The listing builds one solid part. Answer for the finished solid, in the listing's coordinates (mm). Face numbers are marked on the shaded views. A direction names the side the tool comes from. Give positions to 0.01 mm unless a question says otherwise; leave off trailing zeros. Order: outer loops, then holes, each group sorted by start corner. A loop starts at its lowest first (then second) coordinate and runs counter-clockwise, first axis right, second up. Notation, with made-up numbers: (66, 75.5) - (116, 75.5) arc R19 cw to (116, 83.5) - close; hole circle Ø5 at (42, 29). An arc over 180 degrees is marked (long way). Answer as CSV lines item,"result". Start each with the question number.
1. Section D-D on y = 21.75 is taken. Give the vertices of the cut face in (x, z).
2. Section A-A on z = -1 is taken. Give the vertices of the cut face in (x, y).
3. Section B-B on x = 15 is taken. Give the vertices of the cut face in (y, z), and give its area (3 significant figures).
4. Section C-C on z = -10 is taken. Give the vertices of the cut face in (x, y), and give its area (3 significant figures).
5. Flat-ended cylindrical pins translate along their axes: pin 1 (2 mm diameter, centred on x = 15, z = -10, fed in from -Y); pin 2 (1 mm diameter, centred on x = 12, y = 7, fed in from +Z); pin 3 (6 mm diameter, centred on x = 15.5, y = 12.5, fed in from -Z). Find the tip coordinate at first contact, or state that the pin passes through.
6. Consider line 1 along X through (y, z) = (7.35, -10); line 2 along Y through (x, z) = (10.75, -4); line 3 along Z through (x, y) = (15, 23.05). Determine where each line is inside the solid, lowest interval first. Write a range as [from, to].
7. Which of the six approach directions +Z, -Z, +X, -X, +Y, -Y give full straight-line access (tool end or side, diameter ignored) to the marked faces 5 and 6?
8. Determine the mould class of the marked faces 1, 2, 3 and 4 for opening direction Y: +Y half, -Y half, draft (parallel to the pull), parting line (faces both ways), or undercut.
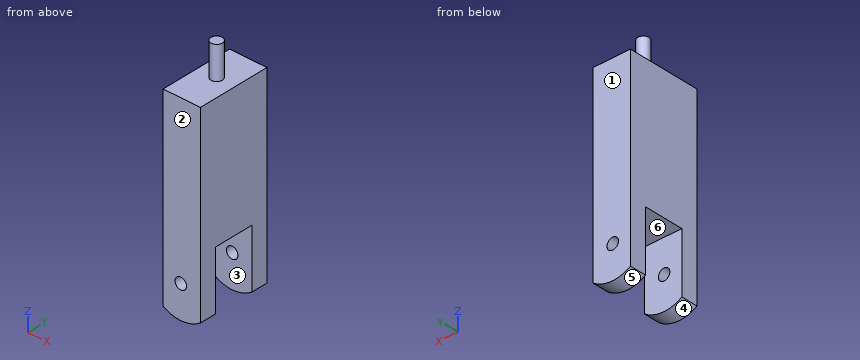
from build123d import *

# Parameters (mm, degrees)
SKETCH3_W            = 30
SKETCH3_H            = 30
BOSS_EXTRUDE1_DEPTH  = 40
CUT_EXTRUDE4_START   = -40
CUT_EXTRUDE4_DEPTH   = 99.309518948
MIRROR5_START        = -40
MIRROR5_COPY_1_DEPTH = 99.309518948
SKETCH9_R            = 1.75
BOSS_EXTRUDE2_DEPTH  = 30
CUT_EXTRUDE5_DEPTH   = 30
SKETCH11_W           = 20
SKETCH11_H           = 12.2
CUT_EXTRUDE6_DEPTH   = 44.5
SKETCH12_R           = 1.75
BOSS_EXTRUDE3_DEPTH  = 10
CUT_EXTRUDE13_DEPTH  = 67
SKETCH16_W           = 6.483229808
SKETCH16_H           = 22.339130026
SKETCH16_W_2         = 7.133382066
CUT_EXTRUDE14_DEPTH  = 67


with BuildPart() as part:
    # Sketch3 → Boss-Extrude1 (new body)
    with BuildSketch(Plane.XY):
        with Locations((15, 15)):
            Rectangle(SKETCH3_W, SKETCH3_H)
    extrude(amount=BOSS_EXTRUDE1_DEPTH)

    # Sketch8 → Cut-Extrude4 (cut)
    with BuildSketch(Plane(origin=(0, 0, 0), x_dir=(-1, 0, 0), z_dir=(0, 0, -1)).offset(CUT_EXTRUDE4_START)):
        Polygon((-77.236567429, -51.703622198), (-30, 17.572977849), (-21.526577959, 30), (25.70998947, 99.276600047), (-112.843210625, 193.749734905), (-215.789767524, 42.769512659), align=None)
    cut_extrude4 = extrude(amount=CUT_EXTRUDE4_DEPTH, mode=Mode.SUBTRACT)

    # Mirror4: Cut-Extrude4 across plane
    add(cut_extrude4.mirror(Plane.ZY.offset(-15)), mode=Mode.SUBTRACT)

    # Mirror5: Cut-Extrude4 across plane
    add(cut_extrude4.mirror(Plane(origin=(0, 15, 0), x_dir=(0, 0, 1), z_dir=(0, -1, 0))), mode=Mode.SUBTRACT)

    # Mirror5 copy 1 sketch → Mirror5 copy 1 (cut)
    with BuildSketch(Plane(origin=(30, 30, 0), x_dir=(1, 0, 0), z_dir=(0, 0, -1)).offset(MIRROR5_START)):
        Polygon((-77.236567429, -51.703622198), (-30, 17.572977849), (-21.526577959, 30), (25.70998947, 99.276600047), (-112.843210625, 193.749734905), (-215.789767524, 42.769512659), align=None)
    extrude(amount=MIRROR5_COPY_1_DEPTH, mode=Mode.SUBTRACT)

    # Sketch9 → Boss-Extrude2 (add)
    with BuildSketch(Plane(origin=(0, 0, 0), x_dir=(1, 0, 0), z_dir=(0, 1, 0))):
        with BuildLine():
            Line((5.769230769, 13.846153846), (0, 0))
            Line((0, 0), (30, 0))
            Line((30, 0), (24.924823528, 11.223878236))
            Line((24.924823528, 11.223878236), (22.474176558, 16.643544594))
            ThreePointArc((22.474176558, 16.643544594), (13.348408887, 19.862669355), (5.769230769, 13.846153846))
        make_face()
        with Locations(Location((15, 10, 0), (0, 0, 270))):
            Circle(SKETCH9_R, mode=Mode.SUBTRACT)
    extrude(amount=BOSS_EXTRUDE2_DEPTH)

    # Sketch10 → Cut-Extrude5 (cut)
    with BuildSketch(Plane.XY):
        Polygon((0, 17.572977849), (8.473422041, 30), (0, 30), align=None)
        Polygon((8.473422041, 0), (0, 0), (0, 12.427022151), align=None)
        Polygon((21.526577959, 0), (30, 12.427022151), (30, 0), align=None)
        Polygon((30, 17.572977849), (21.526577959, 30), (30, 30), align=None)
    extrude(amount=-CUT_EXTRUDE5_DEPTH, mode=Mode.SUBTRACT)

    # Sketch11 → Cut-Extrude6 (cut, symmetric)
    with BuildSketch(Plane(origin=(30, 0, 0), x_dir=(0, 0, -1), z_dir=(1, 0, 0))):
        with Locations((10, 15)):
            Rectangle(SKETCH11_W, SKETCH11_H)
    extrude(amount=CUT_EXTRUDE6_DEPTH, both=True, mode=Mode.SUBTRACT)

    # Sketch12 → Boss-Extrude3 (add)
    with BuildSketch(Plane.XY.offset(40)):
        with Locations(Location((15.321801173, 15.520127928, 0), (0, 0, 180))):
            Circle(SKETCH12_R)
    extrude(amount=BOSS_EXTRUDE3_DEPTH)

    # Sketch15 → Cut-Extrude13 (cut)
    with BuildSketch(Plane.XY.offset(40)):
        Polygon((8.473422041, 30), (5.86162238, 26.169565013), (24.13837762, 26.169565013), (21.526577959, 30), align=None)
        Polygon((30, 17.572977849), (24.220848208, 26.048614609), (24.220848208, 15), (30, 15), align=None)
        Polygon((30, 15), (24.220848208, 15), (24.220848208, 3.951385391), (30, 12.427022151), align=None)
        Polygon((24.13837762, 3.830434987), (5.86162238, 3.830434987), (8.473422041, 0), (21.526577959, 0), align=None)
        Polygon((5.769230769, 3.965935447), (5.815144659, 15), (0, 15), (0, 12.427022151), align=None)
        Polygon((5.815144659, 15), (5.86162238, 26.169565013), (0, 17.572977849), (0, 15), align=None)
    extrude(amount=-CUT_EXTRUDE13_DEPTH, mode=Mode.SUBTRACT)

    # Sketch16 → Cut-Extrude14 (cut)
    with BuildSketch(Plane.XY.offset(40)):
        with Locations((6.355269315, 15)):
            Rectangle(SKETCH16_W, SKETCH16_H)
        with Locations((24.558031714, 15)):
            Rectangle(SKETCH16_W_2, SKETCH16_H)
    extrude(amount=-CUT_EXTRUDE14_DEPTH, mode=Mode.SUBTRACT)


solid = part.part
Checks:
1,outline,"(9.6, -18.41) arc R10 ccw to (20.99, -18.01) - (20.99, 40) - (9.6, 40) - close; hole circle Ø3.5 at (15, -10)"
2,outline,"(9.6, 3.83) - (20.99, 3.83) - (20.99, 8.9) - (9.6, 8.9) - close; (9.6, 21.1) - (20.99, 21.1) - (20.99, 26.17) - (9.6, 26.17) - close"
3,outline,"(3.83, -20) - (8.9, -20) - (8.9, -11.75) - (3.83, -11.75) - close; (3.83, -8.25) - (8.9, -8.25) - (8.9, 0) - (21.1, 0) - (21.1, -8.25) - (26.17, -8.25) - (26.17, 40) - (17.24, 40) - (17.24, 50) - (13.8, 50) - (13.8, 40) - (3.83, 40) - close; (21.1, -20) - (26.17, -20) - (26.17, -11.75) - (21.1, -11.75) - close"
3,area,"1,100 mm²"
4,outline,"(9.6, 3.83) - (13.25, 3.83) - (13.25, 8.9) - (9.6, 8.9) - close; (9.6, 21.1) - (13.25, 21.1) - (13.25, 26.17) - (9.6, 26.17) - close; (16.75, 3.83) - (20.99, 3.83) - (20.99, 8.9) - (16.75, 8.9) - close; (16.75, 21.1) - (20.99, 21.1) - (20.99, 26.17) - (16.75, 26.17) - close"
4,area,"80.0 mm²"
5,pin 1,"passes through"
5,pin 2,"stops at z = 40"
5,pin 3,"stops at z = 0"
6,line 1,"x = [9.6, 13.25], [16.75, 20.99]"
6,line 2,"y = [3.83, 8.9], [21.1, 26.17]"
6,line 3,"z = [-20, -11.75], [-8.25, 40]"
7,face 5,"-Z, +Y, -Y"
7,face 6,"-Z, +X, -X"
8,face 1,"+Y half"
8,face 2,"-Y half"
8,face 3,"undercut"
8,face 4,"draft"
